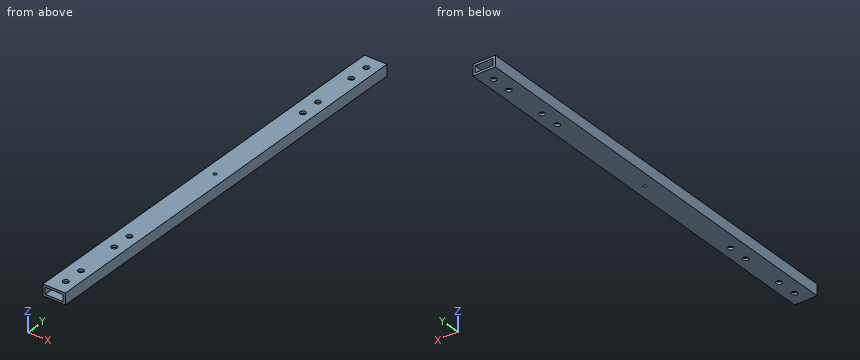
```python
from build123d import *

# Parameters (mm, degrees)
SKETCH_1_W          = 20
SKETCH_1_H          = 10
SKETCH_1_W_2        = 16
SKETCH_1_H_2        = 6
EXTRUDE_1_DEPTH     = 190
SKETCH_2_R          = 2.5
CUT_EXTRUDE_1_DEPTH = 191.525588833
SKETCH_3_R          = 1.5
CUT_EXTRUDE_2_DEPTH = 191.525588833


with BuildPart() as part:
    # 草图1 → 凸台-拉伸1 (new, symmetric)
    with BuildSketch(Plane(origin=(0, 0, 0), x_dir=(1, 0, 0), z_dir=(0, 1, 0))):
        Rectangle(SKETCH_1_W, SKETCH_1_H)
        Rectangle(SKETCH_1_W_2, SKETCH_1_H_2, mode=Mode.SUBTRACT)
    extrude(amount=EXTRUDE_1_DEPTH, both=True)

    # 草图2 → 切除-拉伸1 (cut, through all)
    with BuildSketch(Plane.XY.offset(5)):
        with Locations((1, -177.5)):
            Circle(SKETCH_2_R)
        with Locations((1, -159.7)):
            Circle(SKETCH_2_R)
        with Locations((1, -120.3)):
            Circle(SKETCH_2_R)
        with Locations((1, -102.5)):
            Circle(SKETCH_2_R)
        with Locations(Location((1, 102.5, 0), (0, 0, 180))):
            Circle(SKETCH_2_R)
        with Locations(Location((1, 120.3, 0), (0, 0, 180))):
            Circle(SKETCH_2_R)
        with Locations(Location((1, 159.7, 0), (0, 0, 180))):
            Circle(SKETCH_2_R)
        with Locations(Location((1, 177.5, 0), (0, 0, 180))):
            Circle(SKETCH_2_R)
    extrude(amount=-CUT_EXTRUDE_1_DEPTH, mode=Mode.SUBTRACT)

    # 草图3 → 切除-拉伸2 (cut, through all)
    with BuildSketch(Plane(origin=(0, 0, -5), x_dir=(-1, 0, 0), z_dir=(0, 0, -1))):
        Circle(SKETCH_3_R)
    extrude(amount=-CUT_EXTRUDE_2_DEPTH, mode=Mode.SUBTRACT)


solid = part.part
```
Design review of the part built by this model. Coordinates are the model's own, in mm. Round coordinates to 2 decimals unless told otherwise and drop trailing zeros. Write each loop counter-clockwise with the first axis right and the second up, starting at its lowest first coordinate (ties: lowest second). Pieces come first, ordered by that corner, then holes. Notation, with made-up numbers: (-33, 88.25) -> (-29, 88.25) arc R16 ccw to (-29, 107.25) -> close; hole circle Ø11 at (14, 59.25). An arc over 180 degrees is marked (long way). Answer in a Markdown table with one row per item.
Q1. Take a section at C-C, the plane x = -4.5. State the section outline as (y, z) points, then the cut area to 3 significant figures.
The answers:
| item | result |
|---|---|
| outline | (-190, -5) -> (190, -5) -> (190, -3) -> (-190, -3) -> close; (-190, 3) -> (190, 3) -> (190, 5) -> (-190, 5) -> close |
| area | 1,520 mm² |
Q2. Take a section at B-B, the plane y = -71. State the section outline as (x, z) points.
The answers:
| item | result |
|---|---|
| outline | (-10, -5) -> (10, -5) -> (10, 5) -> (-10, 5) -> close; hole (-8, -3) -> (8, -3) -> (8, 3) -> (-8, 3) -> close |
Q3. Take a section at A-A, the plane z = -1.5. State the section outline as (x, y) points.
The answers:
| item | result |
|---|---|
| outline | (-10, -190) -> (-8, -190) -> (-8, 190) -> (-10, 190) -> close; (8, -190) -> (10, -190) -> (10, 190) -> (8, 190) -> close |
Q4. Clearance check with a flat-ended pin moving along its axis: pin 1 Ø3 at (x, y) = (1, -120.3) entering from -Z. State where the tip first meets the part, or that it passes through.
The answers:
| item | result |
|---|---|
| pin 1 | through |
Q5. To check wall thickness, follow L1, parallel to X at y = -44.5, z = -0.75; L2, parallel to Z at x = 4.25, y = -32; L3, parallel to X at y = 159.7, z = 4.2. State the ranges of each line that lie inside material, in increasing order. Write a range as [from, to].
The answers:
| item | result |
|---|---|
| L1 | [-10, -8], [8, 10] |
| L2 | [-5, -3], [3, 5] |
| L3 | [-10, -1.5], [3.5, 10] |
